Source: CAD feature listing. Evaluate the final solid. Frame: model axes, mm. A direction names the side the tool comes from. Round coordinates to 2 decimals unless told otherwise and drop trailing zeros. Loops run counter-clockwise (first coordinate to the right, second up) from the corner with the lowest first, then second, coordinate; pieces in that order, holes last. Notation, with made-up numbers: (-18.5, 49) -> (31.5, 49) arc R9 cw to (31.5, 56) -> close; hole circle Ø4 at (-18.5, 42.25). An arc over 180 degrees is marked (long way). Write item = value, one per line.
from build123d import *

# Parameters (mm, degrees)
F0_W         = 12
F0_H         = 6
F0_R         = 1.1
F1_DEPTH     = 8
F3_DEPTH     = 5
F4_SIZE      = 0.5
F5_F1_R      = 1
F5_F2_R      = 1
F6_T1_DEPTH  = 13
F6_T3_DEPTH  = 10
F6_T6_ANGLE  = 90
F6_T8_ANGLE  = 90
F6_T10_ANGLE = 90
F6_T12_ANGLE = 90


# Not quite as in the source:
# - a fillet or chamfer that OpenCascade refuses, or shapes differently, is made with other operations: its cross-section is extruded or revolved along the edge and cut away or added


with BuildPart() as f1:
    # F0 (on Top) → F1 (new body)
    with BuildSketch(Plane.XY):
        Rectangle(F0_W, F0_H)
        with Locations((-2.5, 0)):
            Circle(F0_R, mode=Mode.SUBTRACT)
        with BuildLine():
            ThreePointArc((1.05, 0), (2.15, 1.1), (3.25, 0))
            ThreePointArc((3.25, 0), (2.15, -1.1), (1.05, 0))
        make_face(mode=Mode.SUBTRACT)
    extrude(amount=F1_DEPTH)

    # F2 (on Top) → F3 (join)
    with BuildSketch(Plane.XY):
        Polygon((56, -3), (56, 0), (56, 3), (6, 3), (6, 0), (6, -3), align=None)
    extrude(amount=F3_DEPTH)

    # F4
    f4_edges = [f1.edges().sort_by_distance(p)[0] for p in [
        (-3.6, 0, 0),
        (1.05, 0, 0),
    ]]
    chamfer(f4_edges, length=F4_SIZE)

    # F5: fillet of radius 1 on 8 edges, made by hand

    # F5_f1
    f5_f1_edges = [f1.edges().sort_by_distance(p)[0] for p in [
        (6, 0, 5),
    ]]
    fillet(f5_f1_edges, radius=F5_F1_R)

    # F5_f2
    f5_f2_edges = [f1.edges().sort_by_distance(p)[0] for p in [
        (6, -3, 7),
        (6, 3, 7),
        (56, 0, 5),
        (0, -3, 8),
        (6, 0, 8),
        (0, 3, 8),
        (-6, 0, 8),
        (6.2928932188, 3, 5.2928932188),
        (6.2928932188, -3, 5.2928932188),
    ]]
    fillet(f5_f2_edges, radius=F5_F2_R)

    # F6: fillet of radius 2 on 4 edges, made by hand

    # F6_s2 → F6_t1 (cut)
    with BuildSketch(Plane.XY.offset(-5)):
        with BuildLine():
            ThreePointArc((-4, -3), (-5.4142135624, -2.4142135624), (-6, -1))
            Line((-6, -1), (-6, -3))
            Line((-6, -3), (-4, -3))
        make_face()
        with BuildLine():
            ThreePointArc((-6, 1), (-5.4142135624, 2.4142135624), (-4, 3))
            Line((-4, 3), (-6, 3))
            Line((-6, 3), (-6, 1))
        make_face()
    extrude(amount=F6_T1_DEPTH, mode=Mode.SUBTRACT)

    # F6_s4 → F6_t3 (cut)
    with BuildSketch(Plane.XY.offset(-5)):
        with BuildLine():
            ThreePointArc((54, -3), (55.4142135624, -2.4142135624), (56, -1))
            Line((56, -1), (56, -3))
            Line((56, -3), (54, -3))
        make_face()
        with BuildLine():
            ThreePointArc((56, 1), (55.4142135624, 2.4142135624), (54, 3))
            Line((54, 3), (56, 3))
            Line((56, 3), (56, 1))
        make_face()
    extrude(amount=F6_T3_DEPTH, mode=Mode.SUBTRACT)

    # F6_s5 → F6_t6 (revolve, cut)
    with BuildSketch(Plane.XZ.offset(-1)):
        with BuildLine():
            ThreePointArc((55, 5), (55.7071067812, 4.7071067812), (56, 4))
            Line((56, 4), (56, 5))
            Line((56, 5), (55, 5))
        make_face()
    revolve(axis=Axis((54, 1, 5), (0, 0, 1)), revolution_arc=F6_T6_ANGLE, mode=Mode.SUBTRACT)

    # F6_s7 → F6_t8 (revolve, cut)
    with BuildSketch(Plane.YZ.offset(54)):
        with BuildLine():
            ThreePointArc((-2, 5), (-2.7071067812, 4.7071067812), (-3, 4))
            Line((-3, 4), (-3, 5))
            Line((-3, 5), (-2, 5))
        make_face()
    revolve(axis=Axis((54, -1, 5), (0, 0, 1)), revolution_arc=F6_T8_ANGLE, mode=Mode.SUBTRACT)

    # F6_s9 → F6_t10 (revolve, cut)
    with BuildSketch(Plane.YZ.offset(-4)):
        with BuildLine():
            ThreePointArc((2, 8), (2.7071067812, 7.7071067812), (3, 7))
            Line((3, 7), (3, 8))
            Line((3, 8), (2, 8))
        make_face()
    revolve(axis=Axis((-4, 1, 8), (0, 0, 1)), revolution_arc=F6_T10_ANGLE, mode=Mode.SUBTRACT)

    # F6_s11 → F6_t12 (revolve, cut)
    with BuildSketch(Plane.XZ.offset(1)):
        with BuildLine():
            ThreePointArc((-5, 8), (-5.7071067812, 7.7071067812), (-6, 7))
            Line((-6, 7), (-6, 8))
            Line((-6, 8), (-5, 8))
        make_face()
    revolve(axis=Axis((-4, -1, 8), (0, 0, 1)), revolution_arc=F6_T12_ANGLE, mode=Mode.SUBTRACT)


solid = f1.part
1. Section query A-A (y = 0). Return the cut outline in (x, z).
Evaluation:
outline = (-6, 0) -> (-4.1, 0) -> (-3.6, 0.5) -> (-3.6, 8) -> (-5, 8) arc R1 ccw to (-6, 7) -> close; (-1.4, 0.5) -> (-0.9, 0) -> (0.55, 0) -> (1.05, 0.5) -> (1.05, 8) -> (-1.4, 8) -> close; (3.25, 0.5) -> (3.75, 0) -> (56, 0) -> (56, 4) arc R1 ccw to (55, 5) -> (7, 5) arc R1 cw to (6, 6) -> (6, 7) arc R1 ccw to (5, 8) -> (3.25, 8) -> close
2. Section query C-C (x = -2.5). Return the cut outline in (y, z).
Evaluation:
outline = (-3, 0) -> (-1.6, 0) -> (-1.1, 0.5) -> (-1.1, 8) -> (-2, 8) arc R1 ccw to (-3, 7) -> close; (1.1, 0.5) -> (1.6, 0) -> (3, 0) -> (3, 7) arc R1 ccw to (2, 8) -> (1.1, 8) -> close
3. Line query: probe 1 along Y at (x, z) = (-2.5, 5.5); probe 2 along X at (y, z) = (0.25, 2.75); probe 3 along Z at (x, y) = (37.5, 0.25). Output: solid intervals per line, ascending. Write a range as from..to.
Evaluation:
probe_1 = -3..-1.1, 1.1..3
probe_2 = -6..-3.57, -1.43..1.08, 3.22..56
probe_3 = 0..5
4. Section query B-B (z = 3.25). Return the cut outline in (x, y).
Evaluation:
outline = (-6, -1) arc R2 ccw to (-4, -3) -> (54, -3) arc R2 ccw to (56, -1) -> (56, 1) arc R2 ccw to (54, 3) -> (-4, 3) arc R2 ccw to (-6, 1) -> close; hole circle Ø2.2 at (-2.5, 0); hole circle Ø2.2 at (2.15, 0)
5. Mould query, pull axis X, two halves, no side actions, for faces 1 (the face through (25, -3, 2)), 2 (the face through (-1.45, 0.33, 4.2)), 3 (the face through (55.4, -2.43, 1.97)). Classes: released by +X, released by -X, zero draft, split by the parting line, or undercut.
Evaluation:
face_1 = zero draft
face_2 = undercut
face_3 = released by +X
6. Section query D-D (x = 29). Return the cut outline in (y, z).
Evaluation:
outline = (-3, 0) -> (3, 0) -> (3, 4) arc R1 ccw to (2, 5) -> (-2, 5) arc R1 ccw to (-3, 4) -> close
7. Set-up query: faces 4 (the face through (25, 0, 0)), 5 (the face through (31, 0, 5)), 6 (the face through (30.171, -2.715, 4.699)), 7 (the face through (30.171, 2.699, 4.715)), 8 (the face through (-5.699, 0.014, 7.715)). Return all of +Z, -Z, +X, -X, +Y, -Y with unobstructed straight access to the full face (end or side cutting, diameter ignored); none if empty.
Evaluation:
face_4 = -Z, +X, -X, +Y, -Y
face_5 = +Z, +X, +Y, -Y
face_6 = +Z, +X, -Y
face_7 = +Z, +X, +Y
face_8 = +Z, -X, +Y, -Y
8. Contact query for flat-ended pins moving along their axis: pin 1 Ø1.5 at (x, z) = (23, 5.5) entering from +Y; pin 2 Ø2 at (x, y) = (26.5, 0) entering from +Z. Output: stop coordinate, or through.
Evaluation:
pin_1 = 2.66
pin_2 = 5
